The drawing under review shows one solid part. Ordinate dimensions are in mm from its lowest x, y, z. A direction names the side the tool comes from. Round coordinates to 2 decimals unless told otherwise and drop trailing zeros. Write each loop counter-clockwise with the first axis right and the second up, starting at its lowest first coordinate (ties: lowest second). Pieces come first, ordered by that corner, then holes. Notation, with made-up numbers: (-13.75, 77.25) -> (4.25, 77.25) arc R23 cw to (4.25, 103.25) -> close; hole circle Ø1 at (40.5, 35.25). An arc over 180 degrees is marked (long way). Write item = value, one per line. Start each with the question number.
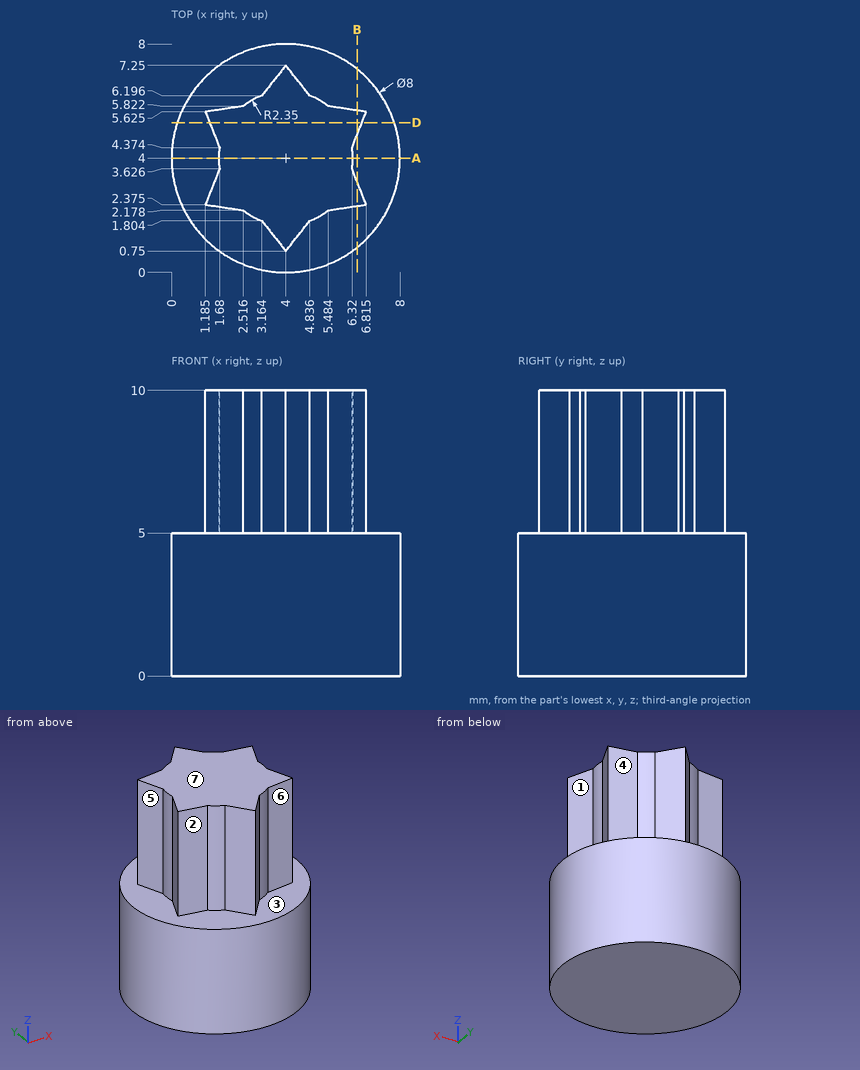
1. Clearance check with a flat-ended pin moving along its axis: pin 1 Ø4 at (y, z) = (5, 6.5) entering from +X. State where the tip first meets the part, or that it passes through.
2. Wall thickness on L1, parallel to Z at x = 4.25, y = 0.5; L2, parallel to X at y = 7, z = 7.75; L3, parallel to Y at x = 5, z = 6.25 (1 decimal): over which ranges is each line inside the solid? List them lowest first. Write a range as from..to.
3. Consider section D-D, the plane y = 5.25. Give the boundary of the cut face in (x, z).
4. Consider section B-B, the plane x = 6.5. Give the boundary of the cut face in (y, z).
5. Consider section A-A, the plane y = 4. Give the boundary of the cut face in (x, z), then the cut area to 3 significant figures.
6. Machinability: for the marked faces 1, 2, 3 and 4, which of the approach directions +Z, -Z, +X, -X, +Y, -Y give a long, thin tool a straight path to every point of the face, cutting with its end or side? Answer none if there is none.
7. Draft analysis for pull direction Y (two halves, no side actions). For the marked faces 5, 6 and 7, state which applies: +Y half, -Y half, draft (parallel to the pull), parting line (faces both ways), or undercut.
Outcome:
q1.pin_1 = 8
q2.L1 = 0..5
q2.L2 = 3.8..4.2
q2.L3 = 1.9..6.1
q3.outline = (0.2, 0) -> (7.8, 0) -> (7.8, 5) -> (6.67, 5) -> (6.67, 10) -> (1.33, 10) -> (1.33, 5) -> (0.2, 5) -> close
q4.outline = (0.88, 0) -> (7.12, 0) -> (7.12, 5) -> (5.67, 5) -> (5.67, 10) -> (4.83, 10) -> (4.83, 5) -> (3.17, 5) -> (3.17, 10) -> (2.33, 10) -> (2.33, 5) -> (0.88, 5) -> close
q5.outline = (0, 0) -> (8, 0) -> (8, 5) -> (6.35, 5) -> (6.35, 10) -> (1.65, 10) -> (1.65, 5) -> (0, 5) -> close
q5.area = 63.5 mm2
q6.face_1 = +Z, +X
q6.face_2 = +Z, -X, -Y
q6.face_3 = +Z
q6.face_4 = +Z, +X, +Y
q7.face_5 = undercut
q7.face_6 = -Y half
q7.face_7 = draft
